Build history of the part. All positions in model axes, mm. A direction names the side the tool comes from. Round coordinates to 2 decimals unless told otherwise and drop trailing zeros. Write each loop counter-clockwise with the first axis right and the second up, starting at its lowest first coordinate (ties: lowest second). Pieces come first, ordered by that corner, then holes. Notation, with made-up numbers: M 59.25,85.25 L 89.25,85.25 A14 cw 89.25,99.25 Z; hole C 43,24.5 d5. An arc over 180 degrees is marked long. Use a Markdown table: item, result.
from build123d import *

# Parameters (mm, degrees)
SKETCH_1_R                       = 58
CUP_PLATE_D116_T4_DEPTH          = 4
SKETCH_2_R                       = 58
SKETCH_2_R_2                     = 55.5
DRIP_SKIRT_OD116_ID111_H10_DEPTH = 10
SKETCH_3_R                       = 2.15
M4_MOVING_MOUNT_CLEARANCE_DEPTH  = 4


with BuildPart() as part:
    # 草图1 → Cup_plate_D116_T4 (new body)
    with BuildSketch(Plane(origin=(0, 0, 0), x_dir=(1, 0, 0), z_dir=(0, 1, 0))):
        with Locations(Location((0, 0, 0), (0, 0, 270))):
            Circle(SKETCH_1_R)
    extrude(amount=CUP_PLATE_D116_T4_DEPTH)

    # 草图2 → Drip_skirt_OD116_ID111_H10 (add)
    with BuildSketch(Plane(origin=(0, 0, 0), x_dir=(1, 0, 0), z_dir=(0, 1, 0))):
        with Locations(Location((0, 0, 0), (0, 0, 270))):
            Circle(SKETCH_2_R)
        with Locations(Location((0, 0, 0), (0, 0, 270))):
            Circle(SKETCH_2_R_2, mode=Mode.SUBTRACT)
    extrude(amount=DRIP_SKIRT_OD116_ID111_H10_DEPTH)

    # 草图3 → M4_moving_mount_clearance (cut)
    with BuildSketch(Plane(origin=(0, 0, 0), x_dir=(1, 0, 0), z_dir=(0, 1, 0))):
        with Locations(Location((-22, 0, 0), (0, 0, 270))):
            Circle(SKETCH_3_R)
        with Locations(Location((-32, 0, 0), (0, 0, 270))):
            Circle(SKETCH_3_R)
    extrude(amount=M4_MOVING_MOUNT_CLEARANCE_DEPTH, mode=Mode.SUBTRACT)


solid = part.part
Q1. Cut at B-B on x = -22. Give the cut face in (y, z).
Response values:
| item | result |
|---|---|
| outline | M 0,-53.67 L 10,-53.67 L 10,-50.95 L 4,-50.95 L 4,-2.15 L 0,-2.15 Z; M 0,2.15 L 4,2.15 L 4,50.95 L 10,50.95 L 10,53.67 L 0,53.67 Z |
Q2. Cut at C-C on y = 8.5. Give the cut face in (x, z), and give its area (3 significant figures).
Response values:
| item | result |
|---|---|
| outline | C 0,0 d116; hole C 0,0 d111 |
| area | 891 mm2 |
Q3. Which spindle directions (+Z, -Z, +X, -X, +Y, -Y) get a long thin tool onto all of the face, cutting with end or side? Do faces 4 (the cylindrical face through (46.798, 6.958, 29.836)), 5 (the cylindrical face through (-24.1, 1.97, -0.47)). Say none if no direction does.
Response values:
| item | result |
|---|---|
| face 4 | +Y |
| face 5 | +Y, -Y |
Q4. Cut at D-D on y = 2.25. Give the cut face in (x, z).
Response values:
| item | result |
|---|---|
| outline | C 0,0 d116; hole C -32,0 d4.3; hole C -22,0 d4.3 |
Q5. Drop flat-ended pins along their axis: P1, Ø6, axis at x = -3, z = 35, coming from the +Y side; P2, Ø1, axis at y = 1.5, z = -40, coming from the -X side; P3, Ø7, axis at x = -32, z = 0, coming from the -Y side; P4, Ø3.5, axis at x = -22, z = 0, coming from the +Y side. Give the stop position or say it passes through.
Response values:
| item | result |
|---|---|
| P1 | stops at y = 4 |
| P2 | stops at x = -42.47 |
| P3 | stops at y = 0 |
| P4 | passes through |
Q6. Cut at A-A on z = 0. Give the cut face in (x, y).
Response values:
| item | result |
|---|---|
| outline | M -58,0 L -34.15,0 L -34.15,4 L -55.5,4 L -55.5,10 L -58,10 Z; M -29.85,0 L -24.15,0 L -24.15,4 L -29.85,4 Z; M -19.85,0 L 58,0 L 58,10 L 55.5,10 L 55.5,4 L -19.85,4 Z |
Q7. Drill centre lines: L1, parallel to X at y = 2.3, z = 0; L2, parallel to X at y = 5.75, z = 0; L3, parallel to Y at x = 49.5, z = -19. Where is each one in solid material? Low to high.
Response values:
| item | result |
|---|---|
| L1 | x = -58 to -34.15, -29.85 to -24.15, -19.85 to 58 |
| L2 | x = -58 to -55.5, 55.5 to 58 |
| L3 | y = 0 to 4 |
Q8. Two-plate mould, pull along X, no slides. Class faces 1 (the cylindrical face through (-22.21, 4.93, 53.58)), 2 (the cylindrical face through (-29.87, 1.97, -0.28)), 3 (the flat face through (1, 0, -1)): +X half, -X half, draft (parallel to the pull), parting line (faces both ways), or undercut.
Response values:
| item | result |
|---|---|
| face 1 | parting line |
| face 2 | undercut |
| face 3 | draft |
